Read the model definition and answer for the solid it produces. Units are mm, in the model's axes. A direction names the side the tool comes from. Coordinates: 2 decimals unless noted, no trailing zeros. Write each loop counter-clockwise with the first axis right and the second up, starting at its lowest first coordinate (ties: lowest second). Pieces come first, ordered by that corner, then holes.
(1) The part is cut by section C-C, the plane z = 5.75. Determine the outline of the cut face in (x, y), and give its area (3 significant figures).
(2) Straight lines are drawn through the part: line 1 along Y through (x, z) = (12, 5.5); line 2 along Z through (x, y) = (0.5, 1.75); line 3 along Y through (x, z) = (13.5, 2.5). For each, find the intervals that lie inside material, in ascending order.
(3) The part is cut by section B-B, the plane x = 13.5. Determine the outline of the cut face in (y, z), and give its area (3 significant figures).
(4) The part is cut by section A-A, the plane y = 0. Determine the outline of the cut face in (x, z).
(5) Determine the mould class of faces 1 (the flat face through (6, 0, 6.5)), 2 (the cylindrical face through (23.5, 0.2, 2.5)), 3 (the flat face through (-1.26, 9.81, 3.2)) for opening direction X: pulls with the +X half, pulls with the -X half, needs draft (parallel to the pull), parting line crosses it, or undercut.
(6) Which of the six approach directions +Z, -Z, +X, -X, +Y, -Y give full straight-line access (tool end or side, diameter ignored) to faces 4 (the flat face through (3.821, 10.068, 2.465)), 5 (the cylindrical face through (16.77, -1.5, 5.74)), 6 (the flat face through (-1.26, -9.81, 3.2))?
(7) Given pin 1 (3 mm diameter, centred on x = 4.5, y = -2.5, fed in from -Z); pin 2 (10 mm diameter, centred on x = 12, y = 1, fed in from +Z); pin 3 (2 mm diameter, centred on y = 5.5, z = 2.5, fed in from -X); pin 4 (1.5 mm diameter, centred on y = 9, z = 4, fed in from -X), each flat-ended and moving along its own axis, determine where each tip first touches the part or whether it passes through.
Autodesk Inventor part; units mm, degrees
ref_plane "YZ Plane" through (0, 0, 0) normal (1, 0, 0) x (0, 1, 0)
ref_plane "XZ Plane" through (0, 0, 0) normal (0, 1, 0) x (-1, 0, 0)
ref_plane "XY Plane" through (0, 0, 0) normal (0, 0, 1) x (1, 0, 0)
ref_plane "作業平面1" through (0, 0, 0) normal (0, 0, 1) x (1, 0, 0)
sketch "スケッチ1" plane through (0, 0, 0) normal (0, 0, 1) x (1, 0, 0)
  arc A0 (9.4, -12.7373) -> (9.4, 12.7373) centre (12, 0) ccw
  circle A1 centre (10.8888, 11) radius 0.8
  circle A2 centre (10.8888, -11) radius 0.8
  circle A3 centre (10.8888, 11) radius 2
  circle A4 centre (10.8888, -11) radius 2
  arc A5 (12.8328, -11.4698) -> (12.8328, 11.4698) centre (12, 0) ccw
  line L0 (9.4, 12.7373) -> (-19.4, 6.8586)
  line L1 (-19.4, -6.8586) -> (9.4, -12.7373)
  line L2 (-1.4086, 10.5311) -> (-1.1086, 9.0614)
  line L3 (-1.1086, 9.0614) -> (8.8914, 11.1026)
  line L4 (-1.4086, -10.5311) -> (-1.1086, -9.0614)
  line L5 (-1.1086, -9.0614) -> (8.8914, -11.1026)
  point P0 (0, 0)
  point P1 (10.1875, -12.873)
  point P2 (11.2013, -12.9754)
  point P3 (11.2013, 12.9754)
  point P4 (10.1875, 12.873)
  dimension "d0" = 4
  dimension "d1" = 1.5
  dimension "d2" = 1.5
  dimension "d3" = 10
extrude "押し出し1" add sketch "スケッチ1" along normal blind 5
sketch "スケッチ2" plane through (0, 0, 5) normal (0, 0, 1) x (1, 0, 0)
  arc A0 (8.8914, 11.1026) -> (12.8328, 11.4698) centre (10.8888, 11) ccw
  arc A1 (12.8328, -11.4698) -> (12.8328, 11.4698) centre (12, 0) ccw
  arc A2 (12.8328, -11.4698) -> (8.8914, -11.1026) centre (10.8888, -11) ccw
  line L0 (8.8914, -11.1026) -> (-1.1086, -9.0614)
  line L1 (-1.1086, -9.0614) -> (-1.4086, -10.5311)
  line L2 (-1.4086, -10.5311) -> (9.4, -12.7373)
  arc A3 (9.4, -12.7373) -> (10.1875, -12.873) centre (12, 0) ccw
  arc A4 (10.1875, -12.873) -> (11.2013, -12.9754) centre (10.8888, -11) ccw
  arc A5 (11.2013, -12.9754) -> (11.2013, 12.9754) centre (12, 0) ccw
  arc A6 (11.2013, 12.9754) -> (10.1875, 12.873) centre (10.8888, 11) ccw
  arc A7 (10.1875, 12.873) -> (9.4, 12.7373) centre (12, 0) ccw
  line L3 (9.4, 12.7373) -> (-1.4086, 10.5311)
  line L4 (-1.4086, 10.5311) -> (-1.1086, 9.0614)
  line L5 (-1.1086, 9.0614) -> (8.8914, 11.1026)
  circle A8 centre (10.8888, -11) radius 0.8
  circle A9 centre (10.8888, 11) radius 0.8
  line L6 (-1.1086, 9.0614) -> (-1.1086, -9.0614)
  circle A10 centre (12, 0) radius 5
  point P0 (0, 0)
  dimension "d6" = 10
extrude "押し出し2" add sketch "スケッチ2" along normal blind 1.5
properties part number "MotorCover"
Computed:
1. outline: (-1.41, -10.53) - (9.4, -12.74) arc R13.02 ccw to (10.19, -12.87) arc R2 ccw to (11.2, -12.98) arc R13 ccw (long way) to (11.2, 12.98) arc R2 ccw to (10.19, 12.87) arc R12.98 ccw to (9.4, 12.74) - (-1.41, 10.53) - (-1.11, 9.06) - (-1.11, -9.06) - close; hole circle Ø10 at (12, 0); hole circle Ø1.6 at (10.89, -11); hole circle Ø1.6 at (10.89, 11)
1. area: 496 mm2
2. line 1: y = -13 to -5, 5 to 13
2. line 2: z = 5 to 6.5
2. line 3: y = -12.91 to -11.4, 11.4 to 12.91
3. outline: (-12.91, 0) - (-11.4, 0) - (-11.4, 5) - (-4.77, 5) - (-4.77, 6.5) - (-12.91, 6.5) - close; (4.77, 5) - (11.4, 5) - (11.4, 0) - (12.91, 0) - (12.91, 6.5) - (4.77, 6.5) - close
3. area: 39.5 mm2
4. outline: (-1.11, 5) - (7, 5) - (7, 6.5) - (-1.11, 6.5) - close; (17, 5) - (23.5, 5) - (23.5, 0) - (25, 0) - (25, 6.5) - (17, 6.5) - close
5. face 1: needs draft
5. face 2: undercut
5. face 3: pulls with the -X half
6. face 4: -Z
6. face 5: +Z, -Z
6. face 6: +Z, -Z, -X
7. pin 1: stops at z = 5
7. pin 2: stops at z = 6.5
7. pin 3: stops at x = 21.49
7. pin 4: stops at x = -1.25
